Geometry: final body of the model. Coordinates: model frame, mm. A direction names the side the tool comes from. Give positions to 0.01 mm unless a question says otherwise; leave off trailing zeros. Order: outer loops, then holes, each group sorted by start corner. A loop starts at its lowest first (then second) coordinate and runs counter-clockwise, first axis right, second up. Notation, with made-up numbers: (73, 28.5) -> (105, 28.5) arc R27 ccw to (105, 63.5) -> close; hole circle Ø1 at (89.5, 59). An arc over 180 degrees is marked (long way). One line per question, with ' | ' between items.
from build123d import *

# Parameters (mm, degrees)
EXTRUDE_1_DEPTH     = 15
SKETCH_2_R          = 2.2
SKETCH_2_R_2        = 10
CUT_EXTRUDE_1_DEPTH = 186.064853497
SKETCH_3_R          = 17.5
CUT_EXTRUDE_2_DEPTH = 186.064853497
FILLET_1_R          = 2


with BuildPart() as part:
    # 草图1 → 凸台-拉伸1 (new body)
    with BuildSketch(Plane.XY):
        with BuildLine():
            Line((1.5, 29.962476533), (161.1, 21.972482791))
            ThreePointArc((161.1, 21.972482791), (182, 0), (161.1, -21.972482791))
            Line((161.1, -21.972482791), (1.5, -29.962476533))
            ThreePointArc((1.5, -29.962476533), (-30, 0), (1.5, 29.962476533))
        make_face()
    extrude(amount=EXTRUDE_1_DEPTH)

    # 草图2 → 切除-拉伸1 (cut, through all)
    with BuildSketch(Plane.XY.offset(15)):
        with Locations((-25, 0)):
            Circle(SKETCH_2_R)
        with Locations((-12.5, 21.650635095)):
            Circle(SKETCH_2_R)
        with Locations((12.5, 21.650635095)):
            Circle(SKETCH_2_R)
        with Locations((25, 0)):
            Circle(SKETCH_2_R)
        with Locations((12.5, -21.650635095)):
            Circle(SKETCH_2_R)
        with Locations((-12.5, -21.650635095)):
            Circle(SKETCH_2_R)
        with Locations((160, 0)):
            Circle(SKETCH_2_R_2)
    extrude(amount=-CUT_EXTRUDE_1_DEPTH, mode=Mode.SUBTRACT)

    # 草图3 → 切除-拉伸2 (cut, through all)
    with BuildSketch(Plane.XY.offset(15)):
        Circle(SKETCH_3_R)
        with BuildLine():
            Line((29.686887248, 18.538843694), (74.686887248, 16.286025909))
            Line((74.686887248, 16.286025909), (54.686887248, -17.287278258))
            Line((54.686887248, -17.287278258), (29.686887248, -18.538843694))
            ThreePointArc((29.686887248, -18.538843694), (35, 0), (29.686887248, 18.538843694))
        make_face()
        Polygon((85.989702062, 15.720177415), (66.684590425, -16.686641834), (111.684590425, -14.433824049), align=None)
        with BuildLine():
            Line((99.713301235, 15.03313812), (142.18397437, 12.906945059))
            ThreePointArc((142.18397437, 12.906945059), (138, 0), (142.18397437, -12.906945059))
            Line((142.18397437, -12.906945059), (124.285212578, -13.803003923))
            Line((124.285212578, -13.803003923), (99.713301235, 15.03313812))
        make_face()
    extrude(amount=-CUT_EXTRUDE_2_DEPTH, mode=Mode.SUBTRACT)

    # 圆角1
    fillet_1_edges = [part.edges().sort_by_distance(p)[0] for p in [
        (124.285212578, -13.803003923, 7.5),
        (99.713301235, 15.03313812, 7.5),
        (142.18397437, 12.906945059, 7.5),
        (142.18397437, -12.906945059, 7.5),
        (85.989702062, 15.720177415, 7.5),
        (111.684590425, -14.433824049, 7.5),
        (66.684590425, -16.686641834, 7.5),
        (74.686887248, 16.286025909, 7.5),
        (54.686887248, -17.287278258, 7.5),
        (29.686887248, -18.538843694, 7.5),
        (29.686887248, 18.538843694, 7.5),
    ]]
    fillet(fillet_1_edges, radius=FILLET_1_R)


solid = part.part
1) Section C-C on y = 0. Count the separate pieces of the cut face and the enclosed holes in it, plus the area to 3 significant figures.
Check result:
separate pieces: 8 | enclosed holes: 0 | area: 1,050 mm^2
2) Material intervals for probe 1 along Y at (x, z) = (105, 3); probe 2 along Y at (x, z) = (-12.5, 11.5); probe 3 along X at (y, z) = (9, 11.75), sorted ascending. Write a range as from..to.
Check result:
probe 1: y = -24.78..-14.77, -6.59..8.83, 14.77..24.78 | probe 2: y = -27.27..-23.85, -19.45..-12.25, 12.25..19.45, 23.85..27.27 | probe 3: x = -28.62..-15.01, 15.01..33.82, 70.35..81.99, 91.72..104.85, 139.93..155.64, 164.36..180.07
3) Set-up query: faces 1 (the cylindrical face through (35, 0, 8)), 2 (the cylindrical face through (182, 0, 7)). Return all of +Z, -Z, +X, -X, +Y, -Y with unobstructed straight access to the full face (end or side cutting, diameter ignored); none if empty.
Check result:
face 1: +Z, -Z | face 2: +Z, -Z, +X
4) Section B-B on x = 12.5. Return loops of the section in (y, z).
Check result:
outline: (-29.41, 0) -> (-23.85, 0) -> (-23.85, 15) -> (-29.41, 15) -> close; (-19.45, 0) -> (-12.25, 0) -> (-12.25, 15) -> (-19.45, 15) -> close; (12.25, 0) -> (19.45, 0) -> (19.45, 15) -> (12.25, 15) -> close; (23.85, 0) -> (29.41, 0) -> (29.41, 15) -> (23.85, 15) -> close
5) Contact query for flat-ended pins moving along their axis: pin 1 Ø3 at (x, z) = (24, 2.5) entering from +Y; pin 2 Ø8 at (y, z) = (21, 5) entering from +X; pin 3 Ø12 at (x, y) = (160, 0) entering from -Z; pin 4 Ø4 at (x, z) = (81, 4) entering from -Y. Output: stop coordinate, or through.
Check result:
pin 1: stops at y = 28.91 | pin 2: stops at x = 173.96 | pin 3: passes through | pin 4: stops at y = -26.08
6) Pull-direction query (X, two-part tool) for faces 3 (the cylindrical face through (-13.887, -10.648, 7.605)), 4 (the flat face through (82.42, -25.91, 7.4)), 5 (the flat face through (77, 7, 0)); classes: +X half, -X half, draft (parallel to the pull), parting line (faces both ways), or undercut.
Check result:
face 3: undercut | face 4: +X half | face 5: draft
7) Section A-A on x = 81.5. Return loops of the section in (y, z), plus the area to 3 significant figures.
Check result:
outline: (-25.96, 0) -> (-15.94, 0) -> (-15.94, 15) -> (-25.96, 15) -> close; (8.18, 0) -> (25.96, 0) -> (25.96, 15) -> (8.18, 15) -> close | area: 417 mm^2
